Source: CAD feature listing. Evaluate the final solid. Frame: model axes, mm. Round coordinates to 2 decimals unless told otherwise and drop trailing zeros. Loops run counter-clockwise (first coordinate to the right, second up) from the corner with the lowest first, then second, coordinate; pieces in that order, holes last.
Item 1: First-contact query: P1, Ø5, axis at x = 42.5, y = 32.5, coming from the +Z side; P2, Ø3, axis at x = 53.5, z = -4.5, coming from the -Y side; P3, Ø3, axis at x = -48, y = 30, coming from the +Z side. Flat tips, straight axial feed; report the tip coordinate or a pass-through.
Item 2: Section query C-C on z = 10. Return loops of the section in (x, y), then the cut area to 3 significant figures.
Item 3: Section query B-B on y = 3. Give the number of separate pieces and of enclosed holes in the cut face, then the cut area to 3 significant figures.
Item 4: Ray query, L1, parallel to X at y = 26, z = 0; L2, parallel to Y at x = 52, z = 0; L3, parallel to X at y = 3.1, z = 0. Return the intervals inside material, ascending.
Item 5: Section query A-A on x = 0. Return loops of the section in (y, z) (3 decimals).
Item 6: Section query D-D on y = 26. Return loops of the section in (x, z) (3 decimals), then the cut area to 3 significant figures.
Item 7: Pull-direction query (Y, two-part tool) for faces 1 (the cylindrical face through (57.34, 20.92, 32.78)), 2 (the flat face through (1, 40.64, -21)), 3 (the cylindrical face through (24.924, 33.974, -49.227)); classes: released by +Y, released by -Y, zero draft, split by the parting line, or undercut.
```python
from build123d import *

# Parameters (mm, degrees)
SKETCH1_R                            = 88.9
BOSS_EXTRUDE1_DEPTH                  = 40.64
SKETCH2_R                            = 20.574
CUT_EXTRUDE1_DEPTH                   = 133.128837125
CUT_EXTRUDE4_DEPTH                   = 133.128837125
CUT_EXTRUDE4_DEPTH_BACK              = 133.128837125
SKETCH3_R                            = 2.032
SKETCH6_R                            = 3.175
CUT_EXTRUDE5_DEPTH                   = 133.128837297
F_1_2_0_5_DIAMETER_HOLE1_D           = 12.7
F_1_2_0_5_DIAMETER_HOLE1_CSINK_D     = 13.97
F_1_2_0_5_DIAMETER_HOLE1_CSINK_ANGLE = 90
CIRPATTERN1_COUNT                    = 6
SKETCH9_W                            = 10.16
SKETCH9_H                            = 5.08


with BuildPart() as part:
    # Sketch1 → Boss-Extrude1 (new body)
    with BuildSketch(Plane(origin=(0, 0, 0), x_dir=(1, 0, 0), z_dir=(0, 1, 0))):
        with Locations(Location((0, 0, 0), (0, 0, 270))):
            Circle(SKETCH1_R)
    extrude(amount=BOSS_EXTRUDE1_DEPTH)

    # Sketch2 → Cut-Extrude1 (cut, through all)
    with BuildSketch(Plane(origin=(0, 40.64, 0), x_dir=(1, 0, 0), z_dir=(0, 1, 0))):
        with Locations(Location((0, 0, 0), (0, 0, 270))):
            Circle(SKETCH2_R)
    extrude(amount=-CUT_EXTRUDE1_DEPTH, mode=Mode.SUBTRACT)

    # Sketch3 → Cut-Extrude4 (cut, two sides: drawn at the far end of the back side and taken through both)
    with BuildSketch(Plane(origin=(0, 0, 0), x_dir=(0, 0, -1), z_dir=(1, 0, 0)).offset(-CUT_EXTRUDE4_DEPTH_BACK)):
        with Locations((0, 21.59)):
            Circle(SKETCH3_R)
    extrude(amount=CUT_EXTRUDE4_DEPTH + CUT_EXTRUDE4_DEPTH_BACK, mode=Mode.SUBTRACT)

    # Sketch6 → Cut-Extrude5 (cut, symmetric)
    with BuildSketch(Plane(origin=(0, 0, 0), x_dir=(0, 1, 0), z_dir=(0.499999999999998, 0, -0.8660254037844398))):
        with Locations(Location((33.02, 0, 0), (0, 0, 270))):
            Circle(SKETCH6_R)
    cut_extrude5 = extrude(amount=CUT_EXTRUDE5_DEPTH, both=True, mode=Mode.SUBTRACT)

    # Mirror1: Cut-Extrude5 across plane
    add(cut_extrude5.mirror(Plane.XY), mode=Mode.SUBTRACT)

    # 1/2 (0.5) Diameter Hole1 (through all)
    with Locations(Plane(origin=(0, 0, 72.39), x_dir=(0, 0, -1), z_dir=(0, -1, 0))):
        with Locations((0, 0)):
            f_1_2_0_5_diameter_hole1 = CounterSinkHole(F_1_2_0_5_DIAMETER_HOLE1_D / 2, F_1_2_0_5_DIAMETER_HOLE1_CSINK_D / 2, counter_sink_angle=F_1_2_0_5_DIAMETER_HOLE1_CSINK_ANGLE)

    # CirPattern1: 1/2 (0.5) Diameter Hole1 ×6 about axis
    cirpattern1_axis = Axis((0, 0, 0), (0, 1, 0))
    for i in range(1, CIRPATTERN1_COUNT):
        add(f_1_2_0_5_diameter_hole1.rotate(cirpattern1_axis, i * 360 / CIRPATTERN1_COUNT), mode=Mode.SUBTRACT)

    # Sketch9 → Cut-Revolve1 (revolve, cut)
    with BuildSketch(Plane.XY, mode=Mode.PRIVATE) as cut_revolve1_sk:
        with Locations((50.8, 2.54)):
            Rectangle(SKETCH9_W, SKETCH9_H)
    revolve(cut_revolve1_sk.sketch.rotate(Axis((0, 40.64, 0), (0, -1, 0)), 90), axis=Axis((0, 40.64, 0), (0, -1, 0)), mode=Mode.SUBTRACT)


solid = part.part
```
Data:
1. P1: stops at z = 79.39
1. P2: stops at y = 5.08
1. P3: stops at z = 75.77
2. outline: (-88.34, 0) - (-54.98, 0) - (-54.98, 5.08) - (-44.61, 5.08) - (-44.61, 0) - (-17.98, 0) - (-17.98, 40.64) - (-88.34, 40.64) - close; (17.98, 0) - (44.61, 0) - (44.61, 5.08) - (54.98, 5.08) - (54.98, 0) - (88.34, 0) - (88.34, 40.64) - (17.98, 40.64) - close
2. area: 5,610 mm2
3. separate pieces: 2
3. enclosed holes: 8
3. area: 19,500 mm2
4. L1: x = -88.9 to -20.57, 20.57 to 88.9
4. L2: y = 5.08 to 19.56, 23.62 to 40.64
4. L3: x = -88.9 to -55.88, -45.72 to -20.57, 20.57 to 45.72, 55.88 to 88.9
5. outline: (0, -88.9) - (40.64, -88.9) - (40.64, -78.74) - (0.635, -78.74) - (0, -79.375) - close; (0, -65.405) - (0.635, -66.04) - (40.64, -66.04) - (40.64, -20.574) - (0, -20.574) - (0, -45.72) - (5.08, -45.72) - (5.08, -55.88) - (0, -55.88) - close; (0, 20.574) - (40.64, 20.574) - (40.64, 66.04) - (0.635, 66.04) - (0, 65.405) - (0, 55.88) - (5.08, 55.88) - (5.08, 45.72) - (0, 45.72) - close; (0, 79.375) - (0.635, 78.74) - (40.64, 78.74) - (40.64, 88.9) - (0, 88.9) - close
6. outline: circle Ø177.8 at (0, 0); hole circle Ø12.7 at (-62.692, -36.195); hole circle Ø12.7 at (-62.692, 36.195); hole circle Ø41.148 at (0, 0); hole circle Ø12.7 at (0, -72.39); hole circle Ø12.7 at (0, 72.39); hole circle Ø12.7 at (62.692, -36.195); hole circle Ø12.7 at (62.692, 36.195)
6. area: 22,700 mm2
7. face 1: zero draft
7. face 2: released by +Y
7. face 3: undercut
